Geometry: final body of the model. Coordinates: model frame, mm. A direction names the side the tool comes from. Give positions to 0.01 mm unless a question says otherwise; leave off trailing zeros. Write each loop counter-clockwise with the first axis right and the second up, starting at its lowest first coordinate (ties: lowest second). Pieces come first, ordered by that corner, then holes. Notation, with made-up numbers: (41, -30.75) -> (85, -30.75) arc R11 ccw to (85, -11.75) -> close; hole circle Ø5 at (8.25, 54.5). An arc over 180 degrees is marked (long way). Answer as a JSON object with one key per item and string values.
from build123d import *

# Parameters (mm, degrees)
SKETCH1_W                   = 60
SKETCH1_H                   = 60
BOSS_EXTRUDE1_DEPTH         = 70
SKETCH2_R                   = 2.3815
CUT_EXTRUDE1_DEPTH          = 71
F_1_4_20_TAPPED_HOLE1_D     = 5.1054
F_1_4_20_TAPPED_HOLE1_DEPTH = 19.05
F_1_4_20_TAPPED_HOLE1_TIP   = 1.533816902


with BuildPart() as part:
    # Sketch1 → Boss-Extrude1 (new body)
    with BuildSketch(Plane(origin=(0, 0, 0), x_dir=(1, 0, 0), z_dir=(0, 1, 0))):
        with Locations((30, 30)):
            Rectangle(SKETCH1_W, SKETCH1_H)
    extrude(amount=BOSS_EXTRUDE1_DEPTH)

    # Sketch2 → Cut-Extrude1 (cut, through all)
    with BuildSketch(Plane.XZ):
        with Locations(Location((10, -30, 0), (0, 0, 270))):  # turned: the seam where the file's is
            Circle(SKETCH2_R)
        with Locations(Location((50, -30, 0), (0, 0, 270))):  # turned: the seam where the file's is
            Circle(SKETCH2_R)
    extrude(amount=-CUT_EXTRUDE1_DEPTH, mode=Mode.SUBTRACT)

    # 1/4-20 Tapped Hole1
    with Locations(Plane(origin=(30, 0, -10), x_dir=(0, 0, -1), z_dir=(0, -1, 0))):
        with Locations((0, 0), (40, 0)):
            Hole(F_1_4_20_TAPPED_HOLE1_D / 2, depth=F_1_4_20_TAPPED_HOLE1_DEPTH)
            with Locations((0, 0, -(F_1_4_20_TAPPED_HOLE1_DEPTH + F_1_4_20_TAPPED_HOLE1_TIP / 2))):  # 118° drill point
                Cone(0, F_1_4_20_TAPPED_HOLE1_D / 2, F_1_4_20_TAPPED_HOLE1_TIP, mode=Mode.SUBTRACT)


solid = part.part
Q1. Mould query, pull axis X, two halves, no side actions, for faces 3 (the flat face through (30, 0, -30)), 4 (the conical face through (30.37, 20.32, -50.24)), 5 (the flat face through (60, 35, -30)). Classes: pulls with the +X half, pulls with the -X half, needs draft (parallel to the pull), parting line crosses it, or undercut.
Values:
{"face 3": "needs draft", "face 4": "undercut", "face 5": "pulls with the +X half"}
Q2. Cut plane A-A (z = -30). Return the cut outline in (x, y), and give its area (3 significant figures).
Values:
{"outline": "(0, 0) -> (7.62, 0) -> (7.62, 70) -> (0, 70) -> close; (12.38, 0) -> (47.62, 0) -> (47.62, 70) -> (12.38, 70) -> close; (52.38, 0) -> (60, 0) -> (60, 70) -> (52.38, 70) -> close", "area": "3,530 mm²"}
Q3. Cut plane B-B (x = 10). Return the cut outline in (y, z), and give its area (3 significant figures).
Values:
{"outline": "(0, -60) -> (70, -60) -> (70, -32.38) -> (0, -32.38) -> close; (0, -27.62) -> (70, -27.62) -> (70, 0) -> (0, 0) -> close", "area": "3,870 mm²"}
Q4. Set-up query: faces 1 (the flat face through (30, 70, -30)), 2 (the cylindrical face through (28.45, 9.66, -52.03)). Return all of +Z, -Z, +X, -X, +Y, -Y with unobstructed straight access to the full face (end or side cutting, diameter ignored); none if empty.
Values:
{"face 1": "+Z, -Z, +X, -X, +Y", "face 2": "-Y"}
Q5. Material intervals for L1, parallel to Z at x = 30, y = 12; L2, parallel to X at y = 32, z = -30; L3, parallel to X at y = 20, z = -29.5, sorted ascending. Write a range as from..to.
Values:
{"L1": "-60..-52.55, -47.45..-12.55, -7.45..0", "L2": "0..7.62, 12.38..47.62, 52.38..60", "L3": "0..7.67, 12.33..47.67, 52.33..60"}
Q6. First-contact query: P1, Ø1, axis at x = 40, y = 49, coming from the +Z side. Flat tip, straight axial feed; report the tip coordinate or a pass-through.
Values:
{"P1": "z = 0"}
